Here's how the part is built. I have some questions about the finished solid (model axes, mm). A direction names the side the tool comes from. Give positions to 0.01 mm unless a question says otherwise; leave off trailing zeros. Write each loop counter-clockwise with the first axis right and the second up, starting at its lowest first coordinate (ties: lowest second). Pieces come first, ordered by that corner, then holes. Notation, with made-up numbers: (-33.5, 79.25) -> (-6.5, 79.25) arc R6 ccw to (-6.5, 83.25) -> close; hole circle Ø8 at (-21.75, 65). An arc over 180 degrees is marked (long way). Use CSV: the item, a comma, the result in double quotes. Start each with the question number.
(1) Suppose I cut it at D-D on x = -64. List the corners of the cut face in (y, z) for me.
(2) I need wall thicknesses on L1, parallel to X at y = -7.5, z = 31; L2, parallel to X at y = 13.5, z = 50; L3, parallel to Z at x = -47, y = -13.25. Which ranges of each line are inside material? Lowest first, please. Write a range as [from, to].
(3) If we mould it in two halves opening along Y, with no side actions, what happens to faces 4 (the flat face through (-32, -15, 31)), 5 (the cylindrical face through (-67.316, -0.182, 1)), 6 (the flat face through (-35, -14, 31)), 7 (the flat face through (-32, 15, 31))? For each: pulls with the +Y half, pulls with the -Y half, needs draft (parallel to the pull), parting line crosses it, or undercut.
(4) Suppose I cut it at C-C on z = 9.5. List the corners of the cut face in (x, y) for me.
(5) Suppose I cut it at A-A on y = 1. List the corners of the cut face in (x, z) for me.
(6) Which directions (+Z, -Z, +X, -X, +Y, -Y) give clear straight access to the entire face, cutting with the end or side of a thin tool? Please do faces 1 (the flat face through (-32.724, -0.21, 29.81)), 2 (the cylindrical face through (-0.6, 0.2, 60.2)), 3 (the flat face through (-34, 0, 0.37)).
(7) Suppose I cut it at B-B on x = -17. List the corners of the cut face in (y, z) for me.
(8) For pin 1 Ø1 at (y, z) = (4, 14) entering from -X; pin 2 Ø3 at (x, y) = (-47, -5.5) entering from +Z; pin 3 Ø8 at (x, y) = (-43.5, 0.5) entering from -Z, each with a flat end and sliding along its axis, tell me the tip position at first contact or that it passes through.
from build123d import *

# Parameters (mm, degrees)
PAD001_DEPTH    = 15
SKETCH003_W     = 93.5093578205
SKETCH003_H     = 26
POCKET_DEPTH    = 0.37
SKETCH004_W     = 69.441960284
SKETCH004_H     = 26
POCKET001_DEPTH = 0.37
FILLET002002_R  = 3
FILLET002003_R  = 0.2
FILLET002004_R  = 1
FILLET002005_R  = 0.2
FILLET002006_R  = 1


with BuildPart() as part:
    # Sketch002 → Pad001 (new body, symmetric)
    with BuildSketch(Plane.XZ):
        Polygon((0, 0), (-70, 0), (0, 62), align=None)
        Polygon((-2, 2.4), (-63.6706055037, 2.4), (-2, 57.0225363033), align=None, mode=Mode.SUBTRACT)
    extrude(amount=PAD001_DEPTH, both=True)

    # Sketch003 (on Face2 of Pad001) → Pocket (cut)
    with BuildSketch(Plane(origin=(-30.7731015554, 0, 34.7438243367), x_dir=(-0.7485881802, 0, -0.6630352453), z_dir=(-0.6630352453, 0, 0.7485881802))):
        with Locations((5.6464937019, 0)):
            Rectangle(SKETCH003_W, SKETCH003_H)
    extrude(amount=-POCKET_DEPTH, mode=Mode.SUBTRACT)

    # Sketch004 (on Face1 of Pocket) → Pocket001 (cut)
    with BuildSketch(Plane(origin=(0, 0, 0), x_dir=(1, 0, 0), z_dir=(0, 0, -1))):
        with Locations((-34.720980142, 0)):
            Rectangle(SKETCH004_W, SKETCH004_H)
    extrude(amount=-POCKET001_DEPTH, mode=Mode.SUBTRACT)

    # Fillet002002
    fillet002002_edges = [part.edges().sort_by_distance(p)[0] for p in [
        (-2, 0, 2.4),
        (-2, 0, 57.022536),
        (-63.670606, 0, 2.4),
    ]]
    fillet(fillet002002_edges, radius=FILLET002002_R)

    # Fillet002003
    fillet002003_edges = [part.edges().sort_by_distance(p)[0] for p in [
        (0, 14, 62),
        (0, -14, 62),
    ]]
    fillet(fillet002003_edges, radius=FILLET002003_R)

    # Fillet002004
    fillet002004_edges = [part.edges().sort_by_distance(p)[0] for p in [
        (0, 0, 61.505736),
    ]]
    fillet(fillet002004_edges, radius=FILLET002004_R)

    # Fillet002005
    fillet002005_edges = [part.edges().sort_by_distance(p)[0] for p in [
        (-70, -14, 0),
        (-70, 14, 0),
    ]]
    fillet(fillet002005_edges, radius=FILLET002005_R)

    # Fillet002006
    fillet002006_edges = [part.edges().sort_by_distance(p)[0] for p in [
        (-69.024218, 0, 0.37),
    ]]
    fillet(fillet002006_edges, radius=FILLET002006_R)


solid = part.part
Geometry says:
1,outline,"(-15, 0) -> (-13, 0) -> (-13, 0.37) -> (13, 0.37) -> (13, 0) -> (15, 0) -> (15, 5.31) -> (13, 5.31) -> (13, 4.82) -> (-13, 4.82) -> (-13, 5.31) -> (-15, 5.31) -> close"
2,L1,"[-34.44, -31.38], [-2, 0]"
2,L2,"[-13.55, -9.93], [-2, 0]"
2,L3,"[0, 2.4], [17.17, 20.37]"
3,face 4,"pulls with the -Y half"
3,face 5,"undercut"
3,face 6,"needs draft"
3,face 7,"pulls with the +Y half"
4,outline,"(-59.27, -15) -> (-55.65, -15) -> (-55.65, 15) -> (-59.27, 15) -> (-59.27, 13) -> (-58.72, 13) -> (-58.72, -13) -> (-59.27, -13) -> close; (-2, -15) -> (0, -15) -> (0, 15) -> (-2, 15) -> close"
5,outline,"(-67.05, 2.12) arc R1 ccw to (-66.39, 0.37) -> (0, 0.37) -> (0, 59.28) arc R1 ccw to (-1.66, 60.03) -> close; hole (-57.75, 7.65) arc R3 ccw to (-55.76, 2.4) -> (-5, 2.4) arc R3 ccw to (-2, 5.4) -> (-2, 50.36) arc R3 ccw to (-6.99, 52.6) -> close"
6,face 1,"+Y, -Y"
6,face 2,"+Z"
6,face 3,"-Z, +X, -X"
7,outline,"(-15, 0) -> (-13, 0) -> (-13, 0.37) -> (13, 0.37) -> (13, 0) -> (15, 0) -> (15, 2.4) -> (-15, 2.4) -> close; (-15, 43.74) -> (15, 43.74) -> (15, 46.94) -> (13, 46.94) -> (13, 46.45) -> (-13, 46.45) -> (-13, 46.94) -> (-15, 46.94) -> close"
8,pin 1,"x = -54.2"
8,pin 2,"z = 21.21"
8,pin 3,"z = 0.37"
